Geometry check sheet. Reference: the model listing, model coordinates, mm. A direction names the side the tool comes from. Coordinates: 2 decimals unless noted, no trailing zeros. Write each loop counter-clockwise with the first axis right and the second up, starting at its lowest first coordinate (ties: lowest second). Pieces come first, ordered by that corner, then holes. Notation, with made-up numbers: (57, 11.5) -> (115, 11.5) arc R17 cw to (115, 24.5) -> close; hole circle Ø8 at (48.5, 8). An arc over 180 degrees is marked (long way). Answer in a Markdown table with one row per item. Add a question column.
1. Cross-section at B-B on x = 16.75. Record the cut outline in (y, z), and give its area (3 significant figures).
2. Scan lines: L1, parallel to X at y = -14, z = 5; L2, parallel to X at y = -8.5, z = -2.5; L3, parallel to Z at x = 15, y = 1.5. Record each from-to range of solid material in increasing order. Write a range as from..to.
3. Cross-section at D-D on y = -12. Record the cut outline in (x, z), and give its area (3 significant figures).
4. Mould release check, pull along Y, two halves, no side actions. Record for faces 5 (the cylindrical face through (14.7, -15.99, 0.13)), 6 (the flat face through (0, 2, 0)): pulls with the +Y half, pulls with the -Y half, needs draft (parallel to the pull), parting line crosses it, or undercut.
5. Cross-section at A-A on z = -11.5. Record the cut outline in (x, y).
6. Depth check by flat-ended pin: P1, Ø1.3, axis at x = 16.5, z = -0.5, coming from the +Y side; P2, Ø2, axis at x = 16.5, z = -1.5, coming from the -Y side; P3, Ø1, axis at x = 7, y = 0.5, coming from the +Z side; P4, Ø2, axis at y = 0, z = 0, coming from the +X side. Enter the tip coordinate at first touch or a pass-through.
7. Set-up check for faces 1 (the cylindrical face through (12.9, 2.8, -0.1)), 2 (the cylindrical face through (18.715, -15.974, 0.133)), 3 (the cylindrical face through (14.685, 0.115, 16.699)), 4 (the flat face through (19, 0, 7)): record each of +Z, -Z, +X, -X, +Y, -Y from which the full face is reachable in a straight line by a thin tool's end or side.
8. Cross-section at C-C on y = 13. Record the cut outline in (x, z), and give its area (3 significant figures).
```python
from build123d import *

# Parameters (mm, degrees)
CORTAR_EXTRUIR1_DEPTH      = 1
CORTAR_EXTRUIR3_DEPTH      = 35
CORTAR_EXTRUIR4_DEPTH      = 24
CORTAR_EXTRUIR5_REACH      = 34.373
CROQUIS6_R                 = 1.8
CORTAR_EXTRUIR6_DEPTH      = 30.24653838
CORTAR_EXTRUIR6_DEPTH_BACK = 3
CROQUIS7_R                 = 2.8
REDONDEO1_R                = 2
REDONDEO2_R                = 1
REDONDEO3_R                = 1


with BuildPart() as part:
    # Croquis1 → Revolución1 (revolve)
    with BuildSketch(Plane.XY, mode=Mode.PRIVATE) as revoluci_n1_sk:
        Polygon((0, 0), (0, 3), (10, 3), (10, 18), (20, 18), (20, 0), align=None)
    revolve(revoluci_n1_sk.sketch.rotate(Axis((-25.36492891, 0, 0), (1, 0, 0)), 90), axis=Axis((-25.36492891, 0, 0), (1, 0, 0)))

    # Croquis2 → Cortar-Extruir1 (cut)
    with BuildSketch(Plane(origin=(20, 0, 0), x_dir=(0, 0, -1), z_dir=(1, 0, 0))):
        with BuildLine():
            Line((-9.183440496, 8.902465622), (-0.902762127, 15.75))
            ThreePointArc((-0.902762127, 15.75), (6.237962948, 0), (-0.902762127, -15.75))
            Line((-0.902762127, -15.75), (-9.50624249, -9.09463967))
            ThreePointArc((-9.50624249, -9.09463967), (-4.229487685, -0.187837691), (-9.183440496, 8.902465622))
        make_face()
    extrude(amount=-CORTAR_EXTRUIR1_DEPTH, mode=Mode.SUBTRACT)

    # Croquis4 → Cortar-Extruir3 (cut)
    with BuildSketch(Plane(origin=(0, 0, -18), x_dir=(-1, 0, 0), z_dir=(0, 0, -1))):
        Polygon((-19, 15.75), (-19, 8.902465622), (-19, -9.09463967), (-19, -15.75), (-19, -16.274754547), (-14.4, -16.274754547), (-14.4, 16.524155196), (-19, 16.524155196), align=None)
    extrude(amount=-CORTAR_EXTRUIR3_DEPTH, mode=Mode.SUBTRACT)

    # Croquis5 → Cortar-Extruir4 (cut)
    with BuildSketch(Plane.XY.offset(18)):
        with BuildLine():
            ThreePointArc((16, -1.341640786), (19, 0), (16, 1.341640786))
            ThreePointArc((16, 1.341640786), (15.44427419, 0), (16, -1.341640786))
        make_face()
    extrude(amount=-CORTAR_EXTRUIR4_DEPTH, mode=Mode.SUBTRACT)

    # Croquis6 → Cortar-Extruir5 (cut, up to next)
    with BuildSketch(Plane.ZY, mode=Mode.PRIVATE) as cortar_extruir5_sk1:
        Circle(CROQUIS6_R)
    cortar_extruir5_tool1 = extrude(cortar_extruir5_sk1.sketch, amount=-CORTAR_EXTRUIR5_REACH, mode=Mode.PRIVATE) & part.part
    add(cortar_extruir5_tool1.solids().sort_by_distance((0, 0, 0))[0], mode=Mode.SUBTRACT)

    # Croquis7 → Cortar-Extruir6 (cut, two sides: drawn at the far end of the back side and taken through both)
    with BuildSketch(Plane(origin=(14.4, 0, 0), x_dir=(0, 0, -1), z_dir=(1, 0, 0)).offset(-CORTAR_EXTRUIR6_DEPTH_BACK)):
        with Locations(Location((0, 0, 0), (0, 0, 270))):
            Circle(CROQUIS7_R)
    extrude(amount=CORTAR_EXTRUIR6_DEPTH + CORTAR_EXTRUIR6_DEPTH_BACK, mode=Mode.SUBTRACT)

    # Redondeo1
    redondeo1_edges = [part.edges().sort_by_distance(p)[0] for p in [
        (19.5, 15.75, 0.902762127),
        (19.5, -15.75, 0.902762127),
        (19.5, -9.09463967, 9.50624249),
        (19.5, 8.902465622, 9.183440496),
    ]]
    fillet(redondeo1_edges, radius=REDONDEO1_R)

    # Redondeo2
    redondeo2_edges = [part.edges().sort_by_distance(p)[0] for p in [
        (19, 16.524155196, 0),
        (14.4, 16.524155196, 0),
        (14.4, -16.274754547, 0),
        (19, -16.274754547, 0),
    ]]
    fillet(redondeo2_edges, radius=REDONDEO2_R)

    # Redondeo3
    redondeo3_edges = [part.edges().sort_by_distance(p)[0] for p in [
        (14.4, 0, 17),
    ]]
    fillet(redondeo3_edges, radius=REDONDEO3_R)


solid = part.part
```
Results found:
| question | item | result |
|---|---|---|
| 1 | outline | (-16.27, -7.69) -> (-16.27, 7.69) arc R18 ccw to start; (-5.92, 17) -> (-1.74, 17) -> (-1.74, 17.92) arc R18 ccw to start; (1.74, 17) -> (5.92, 17) arc R18 ccw to (1.74, 17.92) -> close; (16.52, -7.14) arc R18 ccw to (16.52, 7.14) -> close |
| 1 | area | 36.6 mm^2 |
| 2 | L1 | x = 10..14.4, 19..20 |
| 2 | L2 | x = 10..14.4 |
| 2 | L3 | z = 16.92..17.94 |
| 3 | outline | (10, -13.42) -> (14.4, -13.42) -> (14.4, 13.42) -> (10, 13.42) -> close; (19, -13.42) -> (20, -13.42) -> (20, -2.46) -> (19, -2.46) -> close; (19, 5.75) -> (20, 5.75) -> (20, 13.42) -> (19, 13.42) -> close |
| 3 | area | 137 mm^2 |
| 4 | face 5 | undercut |
| 4 | face 6 | needs draft |
| 5 | outline | (10, -13.85) -> (14.4, -13.85) -> (14.4, 13.85) -> (10, 13.85) -> close; (19, -13.85) -> (20, -13.85) -> (20, 13.85) -> (19, 13.85) -> close |
| 6 | P1 | stops at y = 18 |
| 6 | P2 | stops at y = -17.99 |
| 6 | P3 | stops at z = 3 |
| 6 | P4 | passes through |
| 7 | face 1 | +X |
| 7 | face 2 | +Z, -Z |
| 7 | face 3 | -Z, +Y, -Y |
| 7 | face 4 | -Z |
| 8 | outline | (10, -12.45) -> (14.4, -12.45) -> (14.4, 12.45) -> (10, 12.45) -> close; (19, -12.45) -> (20, -12.45) -> (20, -1.71) -> (19, -1.71) -> close; (19, 4.23) -> (20, 4.23) -> (20, 12.45) -> (19, 12.45) -> close |
| 8 | area | 129 mm^2 |
